```python
from build123d import *

# Parameters (mm, degrees)
BOSS_EXTRUDE1_DEPTH      = 12.7
SKETCH2_R                = 22.225
BOSS_EXTRUDE2_DEPTH      = 76.2
SKETCH3_R                = 20.6375
BOSS_EXTRUDE3_DEPTH      = 254
SKETCH4_R                = 14.2875
CUT_EXTRUDE1_DEPTH       = 203.2
BOSS_EXTRUDE4_DEPTH      = 6.35
BOSS_EXTRUDE4_DEPTH_BACK = 6.35
SKETCH5_W                = 12.7
SKETCH5_H                = 12.7
SKETCH5_R                = 3.175


with BuildPart() as part:
    # Sketch1 → Boss-Extrude1 (new body)
    with BuildSketch(Plane.XY):
        with BuildLine():
            Line((-25.4, 0), (-25.4, 47.625))
            ThreePointArc((-25.4, 47.625), (0, 73.025), (25.4, 47.625))
            Line((25.4, 47.625), (25.4, 0))
            ThreePointArc((25.4, 0), (0, -25.4), (-25.4, 0))
        make_face()
    extrude(amount=BOSS_EXTRUDE1_DEPTH)

    # Sketch2 → Boss-Extrude2 (add)
    with BuildSketch(Plane.XY.offset(12.7)):
        with Locations(Location((0, 47.625, 0), (0, 0, 180))):
            Circle(SKETCH2_R)
    extrude(amount=BOSS_EXTRUDE2_DEPTH)

    # Sketch3 → Boss-Extrude3 (add)
    with BuildSketch(Plane.XY.offset(12.7)):
        Circle(SKETCH3_R)
    extrude(amount=BOSS_EXTRUDE3_DEPTH)

    # Sketch4 → Cut-Extrude1 (cut)
    with BuildSketch(Plane.XY.offset(266.7)):
        Circle(SKETCH4_R)
    extrude(amount=-CUT_EXTRUDE1_DEPTH, mode=Mode.SUBTRACT)

    # Sketch5 → Boss-Extrude4 (add, two sides: drawn at the far end of the back side and taken through both)
    with BuildSketch(Plane(origin=(0, 0, 0), x_dir=(0, 0, -1), z_dir=(1, 0, 0)).offset(-BOSS_EXTRUDE4_DEPTH_BACK)):
        with Locations((6.35, 0)):
            Rectangle(SKETCH5_W, SKETCH5_H)
        with Locations((7.9375, 0)):
            Circle(SKETCH5_R, mode=Mode.SUBTRACT)
    extrude(amount=BOSS_EXTRUDE4_DEPTH + BOSS_EXTRUDE4_DEPTH_BACK)


solid = part.part
```
Work out the finished part from the listing and answer in its coordinate system (mm). A direction names the side the tool comes from. Coordinates: 2 decimals unless noted, no trailing zeros. Loops run counter-clockwise (first coordinate to the right, second up) from the corner with the lowest first, then second, coordinate; pieces in that order, holes last. Notation, with made-up numbers: (48, 25) - (95, 25) arc R20 ccw to (95, 38) - close; hole circle Ø11 at (-23, 60). An arc over 180 degrees is marked (long way). Use a Markdown table: item, result.
Item 1: Find section D-D, the plane x = 17. Determine the outline of the cut face in (y, z).
Evaluation:
| item | result |
|---|---|
| outline | (-18.87, 0) - (66.5, 0) - (66.5, 12.7) - (61.94, 12.7) - (61.94, 88.9) - (33.31, 88.9) - (33.31, 12.7) - (11.7, 12.7) - (11.7, 266.7) - (-11.7, 266.7) - (-11.7, 12.7) - (-18.87, 12.7) - close |
Item 2: Given pin 1 Ø2 at (x, y) = (-3, 17.5) entering from -Z; pin 2 Ø10 at (x, z) = (-0.5, -4) entering from -Y; pin 3 Ø2 at (x, z) = (7.5, 71) entering from +Y; pin 4 Ø10 at (y, z) = (1, -3.5) entering from -X, each flat-ended and moving along its own axis, determine where each tip first touches the part or whether it passes through.
Evaluation:
| item | result |
|---|---|
| pin 1 | stops at z = 0 |
| pin 2 | stops at y = -25.4 |
| pin 3 | stops at y = 68.88 |
| pin 4 | stops at x = -25.4 |
Item 3: For faces 5 (the flat face through (0, 0, 63.5)), 6 (the flat face through (0, 47, 88.9)), 7 (the flat face through (0, 6.35, -6)), 8 (the flat face through (6.35, 2, -5)), 9 (the flat face through (-6.35, 2, -5)), determine the directions among +Z, -Z, +X, -X, +Y, -Y from which every point of the face is accessible in a straight line to the end or side of a thin tool.
Evaluation:
| item | result |
|---|---|
| face 5 | +Z |
| face 6 | +Z, +X, -X, +Y |
| face 7 | -Z, +X, -X, +Y |
| face 8 | -Z, +X, +Y, -Y |
| face 9 | -Z, -X, +Y, -Y |
Item 4: Find section C-C, the plane y = 58. Determine the outline of the cut face in (x, z), and give its area (3 significant figures).
Evaluation:
| item | result |
|---|---|
| outline | (-23.18, 0) - (23.18, 0) - (23.18, 12.7) - (19.65, 12.7) - (19.65, 88.9) - (-19.65, 88.9) - (-19.65, 12.7) - (-23.18, 12.7) - close |
| area | 3,580 mm2 |
Item 5: Find section B-B, the plane z = 232. Determine the outline of the cut face in (x, y) (1 decimal).
Evaluation:
| item | result |
|---|---|
| outline | circle Ø41.3 at (0, 0); hole circle Ø28.6 at (0, 0) |
Item 6: The mould has two halves that part along Y. Classify faces 1 (the cylindrical face through (0.559, -25.394, 6.261)), 2 (the cylindrical face through (-0.56, 73.02, 6.26)), 3 (the flat face through (0, 25, 0)), 4 (the flat face through (2, 24, 12.7)): +Y half, -Y half, draft (parallel to the pull), parting line (faces both ways), or undercut.
Evaluation:
| item | result |
|---|---|
| face 1 | -Y half |
| face 2 | +Y half |
| face 3 | draft |
| face 4 | undercut |
Item 7: Consider probe 1 along Z at (x, y) = (3.5, 2.5); probe 2 along Z at (x, y) = (1.5, 49); probe 3 along X at (y, z) = (-1.5, 72). Determine where each line is inside the solid, lowest interval first. Write a range as from..to.
Evaluation:
| item | result |
|---|---|
| probe 1 | z = -12.7..-9.89, -5.98..63.5 |
| probe 2 | z = 0..88.9 |
| probe 3 | x = -20.58..-14.21, 14.21..20.58 |
